Design review of the part built by this model. Coordinates are the model's own, in mm. Face numbers are marked on the shaded views. Coordinates: 2 decimals unless noted, no trailing zeros. Write each loop counter-clockwise with the first axis right and the second up, starting at its lowest first coordinate (ties: lowest second). Pieces come first, ordered by that corner, then holes. Notation, with made-up numbers: (34.25, 34.5) - (91.25, 34.5) arc R9 cw to (91.25, 49.5) - close; hole circle Ø8 at (35, 73.25). An arc over 180 degrees is marked (long way). One line per item, written item: value.
from build123d import *

# Parameters (mm, degrees)
CIRPATTERN1_COUNT                                   = 6
CSK_FOR_M3_COUNTERSUNK_FLAT_HEAD_SCREW2_D           = 3.2
CSK_FOR_M3_COUNTERSUNK_FLAT_HEAD_SCREW2_CSINK_D     = 6.3
CSK_FOR_M3_COUNTERSUNK_FLAT_HEAD_SCREW2_CSINK_ANGLE = 90
CIRPATTERN2_COUNT                                   = 6


with BuildPart() as part:
    # Sketch1 → Revolve1 (revolve)
    with BuildSketch(Plane.XY, mode=Mode.PRIVATE) as revolve1_sk:
        with BuildLine():
            Line((40, 1), (40, 0))
            Line((40, 0), (46, 0))
            Line((46, 0), (46, 2))
            ThreePointArc((46, 2), (45.121320344, 4.121320344), (43, 5))
            Line((43, 5), (26, 5))
            Line((26, 5), (26, 2))
            Line((26, 2), (39, 2))
            ThreePointArc((39, 2), (39.707106781, 1.707106781), (40, 1))
        make_face()
    revolve(revolve1_sk.sketch.rotate(Axis((0, 96.254, 0), (0, -1, 0)), 90), axis=Axis((0, 96.254, 0), (0, -1, 0)))

    # Sketch3 → CSK for M3 Countersunk Flat Head Screw1 (revolve, cut)
    with BuildSketch(Plane(origin=(43, 5, 0), x_dir=(0, 0, 1), z_dir=(1, 0, 0))):
        Polygon((0, 0), (0, 5), (1.6, 5), (1.6, 4.55), (3.15, 3), (3.15, 0), align=None)
    csk_for_m3_countersunk_flat_head_screw1 = revolve(axis=Axis((43, 11.35, 0), (0, -1, 0)), mode=Mode.SUBTRACT)

    # CirPattern1: CSK for M3 Countersunk Flat Head Screw1 ×6 about axis
    cirpattern1_axis = Axis((0, 0, 0), (0, 1, 0))
    for i in range(1, CIRPATTERN1_COUNT):
        add(csk_for_m3_countersunk_flat_head_screw1.rotate(cirpattern1_axis, i * 360 / CIRPATTERN1_COUNT), mode=Mode.SUBTRACT)

    # CSK for M3 Countersunk Flat Head Screw2 (through all)
    with Locations(Plane(origin=(0, 5, 0), x_dir=(1, 0, 0), z_dir=(0, 1, 0))):
        with Locations((0, 37)):
            csk_for_m3_countersunk_flat_head_screw2 = CounterSinkHole(CSK_FOR_M3_COUNTERSUNK_FLAT_HEAD_SCREW2_D / 2, CSK_FOR_M3_COUNTERSUNK_FLAT_HEAD_SCREW2_CSINK_D / 2, counter_sink_angle=CSK_FOR_M3_COUNTERSUNK_FLAT_HEAD_SCREW2_CSINK_ANGLE)

    # CirPattern2: CSK for M3 Countersunk Flat Head Screw2 ×6 about axis
    cirpattern2_axis = Axis((0, 0, 0), (0, 1, 0))
    for i in range(1, CIRPATTERN2_COUNT):
        add(csk_for_m3_countersunk_flat_head_screw2.rotate(cirpattern2_axis, i * 360 / CIRPATTERN2_COUNT), mode=Mode.SUBTRACT)


solid = part.part
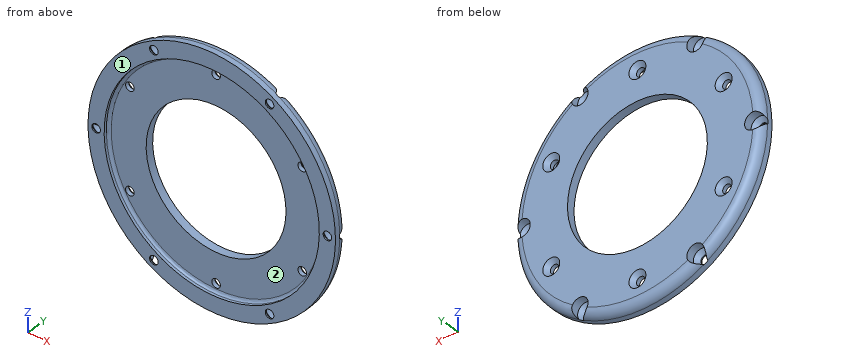
1. Mouldability with a two-part tool opening along X and no side actions: class the marked faces 1 and 2 as released by +X, released by -X, zero draft, split by the parting line, or undercut.
Answer block:
face 1: zero draft
face 2: undercut
2. Consider section A-A, the plane x = 0. Write out the cut boundary in (y, z), then the cut area to 3 significant figures.
Answer block:
outline: (0, -46) - (2, -46) arc R3 ccw to (5, -43) - (5, -40.15) - (3.45, -38.6) - (2, -38.6) - (2, -39) arc R1 cw to (1, -40) - (0, -40) - close; (0, 40) - (1, 40) arc R1 cw to (2, 39) - (2, 38.6) - (3.45, 38.6) - (5, 40.15) - (5, 43) arc R3 ccw to (2, 46) - (0, 46) - close; (2, -35.4) - (3.45, -35.4) - (5, -33.85) - (5, -26) - (2, -26) - close; (2, 26) - (5, 26) - (5, 33.85) - (3.45, 35.4) - (2, 35.4) - close
area: 117 mm^2
3. Insertion check: pin 1 Ø2.5 at (x, z) = (-32.04, -18.5) entering from -Y; pin 2 Ø1 at (y, z) = (3, -5) entering from +X; pin 3 Ø5 at (x, z) = (14, -31) entering from -Y; pin 4 Ø5 at (x, z) = (-43, 0) entering from +Y. Each pin has a flat end and moves straight along its axis. Give the tip position at first contact, or say it passes through.
Answer block:
pin 1: passes through
pin 2: stops at x = 45.7
pin 3: stops at y = 2
pin 4: stops at y = 1.35
4. Wall thickness on line 1 along X through (y, z) = (0.3, 0); line 2 along X through (y, z) = (2.6, -37); line 3 along Z through (x, y) = (32, 3.9): over which ranges is each line inside the solid? List them lowest first.
Answer block:
line 1: x = -46 to -44.6, -41.4 to -40, 40 to 41.4, 44.6 to 46
line 2: x = -27.23 to -24.64, -18.36 to -1.6, 1.6 to 18.36, 24.64 to 27.23
line 3: z = -32.09 to -20.55, -16.45 to 16.45, 20.55 to 32.09
